```python
from build123d import *

# Parameters (mm, degrees)
EXTRUDE_1_DEPTH     = 12.5
EXTRUDE_START       = 5
EXTRUDE_3_DEPTH     = 5
EXTRUDE_4_DEPTH     = 7
EXTRUDE_START_2     = -45
EXTRUDE_5_DEPTH     = 45
CUT_EXTRUDE_1_DEPTH = 45


with BuildPart() as part:
    # 草图1 → 凸台-拉伸1 (new, symmetric)
    with BuildSketch(Plane(origin=(0, 0, 0), x_dir=(1, 0, 0), z_dir=(0, 1, 0))):
        with BuildLine():
            Line((18.5, 18.648056199), (18.5, 25))
            Line((18.5, 25), (-18.5, 25))
            Line((-18.5, 25), (-18.5, 7.5))
            Line((-18.5, 7.5), (-31.5, 7.5))
            Line((-31.5, 7.5), (-31.5, -7.5))
            Line((-31.5, -7.5), (-18.5, -7.5))
            Line((-18.5, -7.5), (-18.5, -25))
            Line((-18.5, -25), (18.5, -25))
            Line((18.5, -25), (18.5, -18.648056199))
            ThreePointArc((18.5, -18.648056199), (12, 0), (18.5, 18.648056199))
        make_face()
    extrude(amount=EXTRUDE_1_DEPTH, both=True)

    # 草图2 → 凸台-拉伸3 (add)
    with BuildSketch(Plane(origin=(0, 4, 0), x_dir=(1, 0, 0), z_dir=(0, 1, 0)).offset(EXTRUDE_START)):
        with BuildLine():
            Line((18.5, 23.648056199), (29.5, 23.648056199))
            Line((29.5, 23.648056199), (29.5, 18.648056199))
            ThreePointArc((29.5, 18.648056199), (26.175718971, 13.433463712), (23.991255863, 7.648056199))
            Line((23.991255863, 7.648056199), (12.991255863, 7.648056199))
            ThreePointArc((12.991255863, 7.648056199), (15.175718971, 13.433463712), (18.5, 18.648056199))
            Line((18.5, 18.648056199), (18.5, 23.648056199))
        make_face()
        with BuildLine():
            Line((12.991255863, -7.648056199), (23.991255863, -7.648056199))
            ThreePointArc((23.991255863, -7.648056199), (26.175718971, -13.433463712), (29.5, -18.648056199))
            Line((29.5, -18.648056199), (29.5, -23.648056199))
            Line((29.5, -23.648056199), (18.5, -23.648056199))
            Line((18.5, -23.648056199), (18.5, -18.648056199))
            ThreePointArc((18.5, -18.648056199), (15.175718971, -13.433463712), (12.991255863, -7.648056199))
        make_face()
    extrude_3 = extrude(amount=-EXTRUDE_3_DEPTH)

    # 镜向1: 凸台-拉伸3 across plane
    add(extrude_3.mirror(Plane.ZX))

    # 草图3 → 凸台-拉伸4 (add)
    with BuildSketch(Plane(origin=(0, 12.5, 0), x_dir=(1, 0, 0), z_dir=(0, 1, 0))):
        with BuildLine():
            Line((-13.170764362, 6.5), (-18.170764362, 6.5))
            ThreePointArc((-18.170764362, 6.5), (-24.670764362, 0), (-18.170764362, -6.5))
            Line((-18.170764362, -6.5), (-13.170764362, -6.5))
            ThreePointArc((-13.170764362, -6.5), (-6.670764362, 0), (-13.170764362, 6.5))
        make_face()
    extrude(amount=EXTRUDE_4_DEPTH)

    # 草图5 → 凸台-拉伸5 (add)
    with BuildSketch(Plane(origin=(0, 19.5, 0), x_dir=(1, 0, 0), z_dir=(0, 1, 0)).offset(EXTRUDE_START_2)):
        with BuildLine():
            Line((-18.170764362, 6.5), (-13.170764362, 6.5))
            ThreePointArc((-13.170764362, 6.5), (-6.670764362, 0), (-13.170764362, -6.5))
            Line((-13.170764362, -6.5), (-18.170764362, -6.5))
            ThreePointArc((-18.170764362, -6.5), (-24.670764362, 0), (-18.170764362, 6.5))
        make_face()
    extrude(amount=EXTRUDE_5_DEPTH)

    # 草图6 → 切除-拉伸1 (cut)
    with BuildSketch(Plane(origin=(0, 19.5, 0), x_dir=(1, 0, 0), z_dir=(0, 1, 0))):
        with BuildLine():
            Line((-18.170764362, 4), (-13.170764362, 4))
            ThreePointArc((-13.170764362, 4), (-9.170764362, 0), (-13.170764362, -4))
            Line((-13.170764362, -4), (-18.170764362, -4))
            ThreePointArc((-18.170764362, -4), (-22.170764362, 0), (-18.170764362, 4))
        make_face()
    extrude(amount=-CUT_EXTRUDE_1_DEPTH, mode=Mode.SUBTRACT)


solid = part.part
```
Verification items for the finished model (mm, model axes). A direction names the side the tool comes from. Round coordinates to 2 decimals unless told otherwise and drop trailing zeros. Order: outer loops, then holes, each group sorted by start corner. A loop starts at its lowest first (then second) coordinate and runs counter-clockwise, first axis right, second up.
1) Cross-section at A-A, the plane z = 0. Record the cut outline in (x, y), plus the area to 4 significant figures.
Geometry says:
outline: (-31.5, -12.5) - (-24.67, -12.5) - (-24.67, -25.5) - (-22.17, -25.5) - (-22.17, 19.5) - (-24.67, 19.5) - (-24.67, 12.5) - (-31.5, 12.5) - close; (-9.17, -25.5) - (-6.67, -25.5) - (-6.67, -12.5) - (12, -12.5) - (12, 12.5) - (-6.67, 12.5) - (-6.67, 19.5) - (-9.17, 19.5) - close
area: 862.5 mm2
2) Cross-section at C-C, the plane x = 21. Record the cut outline in (y, z), plus the area to 3 significant figures.
Geometry says:
outline: (-9, -23.65) - (-4, -23.65) - (-4, -7.65) - (-9, -7.65) - close; (-9, 7.65) - (-4, 7.65) - (-4, 23.65) - (-9, 23.65) - close; (4, -23.65) - (9, -23.65) - (9, -7.65) - (4, -7.65) - close; (4, 7.65) - (9, 7.65) - (9, 23.65) - (4, 23.65) - close
area: 320 mm2
3) Draft check along Y on faces 4 (the flat face through (-15.5, -25.5, 4.2)), 5 (the flat face through (18.5, 0, 23)), 6 (the flat face through (24, 7, 23.648)), 7 (the flat face through (21, 4, -16)). Enter one of: +Y half, -Y half, draft (parallel to the pull), parting line (faces both ways), or undercut.
Geometry says:
face 4: -Y half
face 5: undercut
face 6: draft
face 7: undercut
4) Cross-section at B-B, the plane y = 14.5. Record the cut outline in (x, z), plus the area to 3 significant figures.
Geometry says:
outline: (-18.17, -6.5) - (-13.17, -6.5) arc R6.5 ccw to (-13.17, 6.5) - (-18.17, 6.5) arc R6.5 ccw to start; hole (-18.17, -4) - (-13.17, -4) arc R4 ccw to (-13.17, 4) - (-18.17, 4) arc R4 ccw to start
area: 107 mm2
5) Depth check by flat-ended pin: pin 1 (1.5 mm diameter, centred on x = -16.5, y = 14.5, fed in from +Z); pin 2 (6.5 mm diameter, centred on x = -26.5, y = 1.5, fed in from +Z); pin 3 (1.5 mm diameter, centred on x = 23, y = -6.5, fed in from -Z). Enter the tip coordinate at first touch or a pass-through.
Geometry says:
pin 1: stops at z = 6.5
pin 2: stops at z = 7.5
pin 3: stops at z = -23.65
6) Material ranges on line 1 (Y direction, x = 15.5, z = -13.5); line 2 (Z direction, x = -18, y = -13); line 3 (Y direction, x = -3.5, z = -1), recorded low to high.
Geometry says:
line 1: y = -9 to -4, 4 to 9
line 2: z = -6.5 to -4, 4 to 6.5
line 3: y = -12.5 to 12.5
7) Cross-section at D-D, the plane z = -5. Record the cut outline in (x, y), plus the area to 3 significant figures.
Geometry says:
outline: (-31.5, -12.5) - (-22.32, -12.5) - (-22.32, -25.5) - (-9.02, -25.5) - (-9.02, -12.5) - (12.42, -12.5) - (12.42, 12.5) - (-9.02, 12.5) - (-9.02, 19.5) - (-22.32, 19.5) - (-22.32, 12.5) - (-31.5, 12.5) - close
area: 1,360 mm2
8) Tool access check on faces 1 (the cylindrical face through (-24.67, -19.09, 0.14)), 2 (the cylindrical face through (-6.672, -19.091, -0.143)), 3 (the flat face through (18, 7, 7.648)). Record the directions out of +Z, -Z, +X, -X, +Y, -Y that give a thin tool (end or side, any length) a straight path to the whole face; none if there is none.
Geometry says:
face 1: -X, -Y
face 2: +X, -Y
face 3: +X, +Y, -Y
